Drawing for the job (mm, zero at the part's lowest x, y, z). A direction names the side the tool comes from. Round coordinates to 2 decimals unless told otherwise and drop trailing zeros. Loops run counter-clockwise (first coordinate to the right, second up) from the corner with the lowest first, then second, coordinate; pieces in that order, holes last. Notation, with made-up numbers: M 68,-28.5 L 110,-28.5 A18 ccw 110,-20.5 Z; hole C 7.5,-38.5 d9. An arc over 180 degrees is marked long. Use a Markdown table: item, result. Add a question column.
Q1. Cut at A-A (z = 10.16). Give the cut face in (x, y) (1 decimal), plus the area to 3 significant figures.
Q2. Mould opens along X. For the marked faces 3, 4 and 5 say: +X half, -X half, draft (parallel to the pull), parting line (faces both ways), or undercut.
Q3. Cut at B-B (y = 8.5). State how many separate pieces and enclosed holes the cut face has, plus the area to 3 significant figures.
Q4. Cut at D-D (z = 19.5). Give the cut face in (x, y) (3 decimals).
Q5. Cut at C-C (x = 43.5). Give the cut face in (y, z).
Q6. Probe line 1 (X direction, y = 1.75, z = 8) (3 decimals); line 2 (Z direction, x = 37, y = 1); line 3 (Z direction, x = 58.5, y = 2.5). List the from-to ranges inside material, lowest first. Write a range as from..to.
Q7. Tool access for the marked faces 1 and 2: list every direction of +Z, -Z, +X, -X, +Y, -Y with a clear straight run to the whole face (end or side of a thin tool).
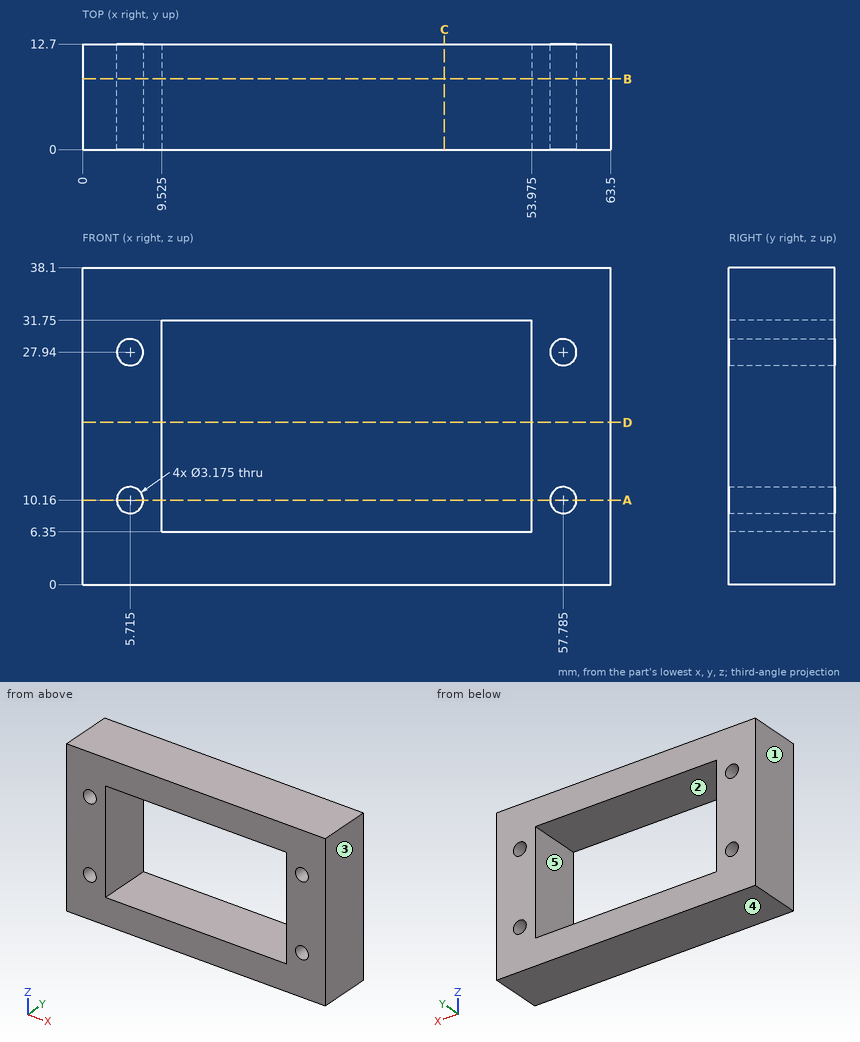
Checked values:
| question | item | result |
|---|---|---|
| 1 | outline | M 0,0 L 4.1,0 L 4.1,12.7 L 0,12.7 Z; M 7.3,0 L 9.5,0 L 9.5,12.7 L 7.3,12.7 Z; M 54,0 L 56.2,0 L 56.2,12.7 L 54,12.7 Z; M 59.4,0 L 63.5,0 L 63.5,12.7 L 59.4,12.7 Z |
| 1 | area | 161 mm^2 |
| 2 | face 3 | +X half |
| 2 | face 4 | draft |
| 2 | face 5 | undercut |
| 3 | separate pieces | 1 |
| 3 | enclosed holes | 5 |
| 3 | area | 1,260 mm^2 |
| 4 | outline | M 0,0 L 9.525,0 L 9.525,12.7 L 0,12.7 Z; M 53.975,0 L 63.5,0 L 63.5,12.7 L 53.975,12.7 Z |
| 5 | outline | M 0,0 L 12.7,0 L 12.7,6.35 L 0,6.35 Z; M 0,31.75 L 12.7,31.75 L 12.7,38.1 L 0,38.1 Z |
| 6 | line 1 | x = 0..9.525, 53.975..63.5 |
| 6 | line 2 | z = 0..6.35, 31.75..38.1 |
| 6 | line 3 | z = 0..8.74, 11.58..26.52, 29.36..38.1 |
| 7 | face 1 | +Z, -Z, -X, +Y, -Y |
| 7 | face 2 | +Y, -Y |
